Part model, mm, in its own coordinate system. Round coordinates to 2 decimals unless told otherwise and drop trailing zeros. Write each loop counter-clockwise with the first axis right and the second up, starting at its lowest first coordinate (ties: lowest second). Pieces come first, ordered by that corner, then holes. Notation, with made-up numbers: (-39, 72) -> (-31, 72) arc R16 ccw to (-31, 81) -> close; hole circle Ø8 at (39, -9.75). An arc over 180 degrees is marked (long way). Return JSON: item names as keys, results as strings. Group by question number.
(1) Drop flat-ended pins along their axis: pin 1 Ø12 at (x, y) = (12, 53) entering from -Z; pin 2 Ø5.5 at (x, y) = (-20, -97) entering from -Z. Give the stop position or say it passes through.
(2) Saw through at A-A (x = -20). List the corners of the cut face in (y, z), plus the area to 3 significant figures.
(3) Drill centre lines: L1, parallel to Y at x = 20, z = 2.5; L2, parallel to Y at x = 1.5, z = 3.5; L3, parallel to Y at x = 17, z = 3. Where is each one in solid material? Low to high. Write a range as from..to.
(4) Saw through at C-C (z = 3). State how many separate pieces and enclosed holes the cut face has, plus the area to 3 significant figures.
(5) Saw through at B-B (y = -97). List the corners of the cut face in (x, z), plus the area to 3 significant figures.
(6) Mould opens along Y. For faces 1 (the flat face through (38, -1, 3)), 2 (the flat face through (-35, 103, 3)), 3 (the cylindrical face through (-18.226, 99.783, 3.042)) say: +Y half, -Y half, draft (parallel to the pull), parting line (faces both ways), or undercut.
from build123d import *

# Parameters (mm, degrees)
SKETCH_1_W             = 76
SKETCH_1_H             = 210
EXTRUDE_1_DEPTH        = 6
SKETCH_2_R             = 3.3
CUT_EXTRUDE_1_DEPTH    = 112.825757319
CHAMFER_2_SIZE         = 5
CHAMFER_1_SIZE         = 1
HOLE_WIZARD_M4_1_D     = 3.3
HOLE_WIZARD_M4_1_DEPTH = 10.1
HOLE_WIZARD_M4_1_TIP   = 0.991420021
HOLE_WIZARD_M3_1_D     = 2.5
HOLE_WIZARD_M3_1_DEPTH = 7.5
HOLE_WIZARD_M3_1_TIP   = 0.751075774
SKETCH_7_R             = 12.5
CUT_EXTRUDE_2_DEPTH    = 112.825757319
SKETCH_8_R             = 12.5
CUT_EXTRUDE_3_DEPTH    = 112.825757319
CHAMFER_3_SIZE         = 1


with BuildPart() as part:
    # 草图1 → 凸台-拉伸1 (new body)
    with BuildSketch(Plane.XY):
        Rectangle(SKETCH_1_W, SKETCH_1_H)
    extrude(amount=EXTRUDE_1_DEPTH)

    # 草图2 → 切除-拉伸1 (cut, through all)
    with BuildSketch(Plane.XY.offset(6)):
        with Locations((-20, 97)):
            Circle(SKETCH_2_R)
        with Locations((20, 97)):
            Circle(SKETCH_2_R)
        with Locations((-20, -97)):
            Circle(SKETCH_2_R)
        with Locations((20, -97)):
            Circle(SKETCH_2_R)
    extrude(amount=-CUT_EXTRUDE_1_DEPTH, mode=Mode.SUBTRACT)

    # 倒角2
    chamfer_2_edges = [part.edges().sort_by_distance(p)[0] for p in [
        (38, -105, 3),
        (-38, -105, 3),
        (-38, 105, 3),
        (38, 105, 3),
    ]]
    chamfer(chamfer_2_edges, length=CHAMFER_2_SIZE)

    # 倒角1
    chamfer_1_edges = [part.edges().sort_by_distance(p)[0] for p in [
        (0, -105, 0),
        (0, -105, 6),
        (38, 0, 0),
        (-38, 0, 0),
        (0, 105, 0),
        (35.5, 102.5, 0),
        (-35.5, 102.5, 0),
        (35.5, -102.5, 0),
        (-35.5, -102.5, 0),
        (-38, 0, 6),
        (38, 0, 6),
        (0, 105, 6),
        (35.5, 102.5, 6),
        (-35.5, 102.5, 6),
        (35.5, -102.5, 6),
        (-35.5, -102.5, 6),
    ]]
    chamfer(chamfer_1_edges, length=CHAMFER_1_SIZE)

    # M4 螺纹孔1
    with Locations(Plane(origin=(0, 0, 0), x_dir=(-1, 0, 0), z_dir=(0, 0, -1))):
        with Locations((-16, 14), (16, 14), (16, -69), (-16, -69)):
            Hole(HOLE_WIZARD_M4_1_D / 2, depth=HOLE_WIZARD_M4_1_DEPTH)
            with Locations((0, 0, -(HOLE_WIZARD_M4_1_DEPTH + HOLE_WIZARD_M4_1_TIP / 2))):  # 118° drill point
                Cone(0, HOLE_WIZARD_M4_1_D / 2, HOLE_WIZARD_M4_1_TIP, mode=Mode.SUBTRACT)

    # M3 螺纹孔1
    with Locations(Plane(origin=(0, 0, 0), x_dir=(-1, 0, 0), z_dir=(0, 0, -1))):
        with Locations((0, 58), (0, 88)):
            Hole(HOLE_WIZARD_M3_1_D / 2, depth=HOLE_WIZARD_M3_1_DEPTH)
            with Locations((0, 0, -(HOLE_WIZARD_M3_1_DEPTH + HOLE_WIZARD_M3_1_TIP / 2))):  # 118° drill point
                Cone(0, HOLE_WIZARD_M3_1_D / 2, HOLE_WIZARD_M3_1_TIP, mode=Mode.SUBTRACT)

    # 草图7 → 切除-拉伸2 (cut, through all)
    with BuildSketch(Plane(origin=(0, 0, 0), x_dir=(-1, 0, 0), z_dir=(0, 0, -1))):
        with Locations((0, 73)):
            Circle(SKETCH_7_R)
    extrude(amount=-CUT_EXTRUDE_2_DEPTH, mode=Mode.SUBTRACT)

    # 草图8 → 切除-拉伸3 (cut, through all)
    with BuildSketch(Plane(origin=(0, 0, 0), x_dir=(-1, 0, 0), z_dir=(0, 0, -1))):
        with Locations((-0.670705331, -27.019604997)):
            Circle(SKETCH_8_R)
    extrude(amount=-CUT_EXTRUDE_3_DEPTH, mode=Mode.SUBTRACT)

    # 倒角3
    chamfer_3_edges = [part.edges().sort_by_distance(p)[0] for p in [
        (12.5, 73, 6),
        (12.5, 73, 0),
        (13.170705331, -27.019604997, 6),
        (13.170705331, -27.019604997, 0),
    ]]
    chamfer(chamfer_3_edges, length=CHAMFER_3_SIZE)


solid = part.part
Computed values:
{
 "1": {"pin 1": "z = 0", "pin 2": "through"},
 "2": {"outline": "(-105, 1) -> (-104, 0) -> (-100.3, 0) -> (-100.3, 6) -> (-104, 6) -> (-105, 5) -> close; (-93.7, 0) -> (93.7, 0) -> (93.7, 6) -> (-93.7, 6) -> close; (100.3, 0) -> (104, 0) -> (105, 1) -> (105, 5) -> (104, 6) -> (100.3, 6) -> close", "area": "1,180 mm2"},
 "3": {"L1": "-105..-100.3, -93.7..93.7, 100.3..105", "L2": "-105..-39.49, -14.55..60.59, 85.41..105", "L3": "-105..-98.37, -95.63..-70.31, -67.69..12.69, 15.31..95.63, 98.37..105"},
 "4": {"separate pieces": "1", "enclosed holes": "12", "area": "14,700 mm2"},
 "5": {"outline": "(-38, 1) -> (-37, 0) -> (-23.3, 0) -> (-23.3, 6) -> (-37, 6) -> (-38, 5) -> close; (-16.7, 0) -> (16.7, 0) -> (16.7, 6) -> (-16.7, 6) -> close; (23.3, 0) -> (37, 0) -> (38, 1) -> (38, 5) -> (37, 6) -> (23.3, 6) -> close", "area": "375 mm2"},
 "6": {"face 1": "draft", "face 2": "+Y half", "face 3": "undercut"}
}
